Input: dimensioned drawing with shaded views. Units: mm. Origin: part minimum x, y, z. A direction names the side the tool comes from. Coordinates: 2 decimals unless noted, no trailing zeros. Order: outer loops, then holes, each group sorted by start corner. A loop starts at its lowest first (then second) coordinate and runs counter-clockwise, first axis right, second up. Notation, with made-up numbers: (-1.75, 70.25) -> (12.25, 70.25) arc R22 cw to (12.25, 91.25) -> close; hole circle Ø7 at (-17, 50). An arc over 180 degrees is marked (long way). Answer as CSV lines item,"result".
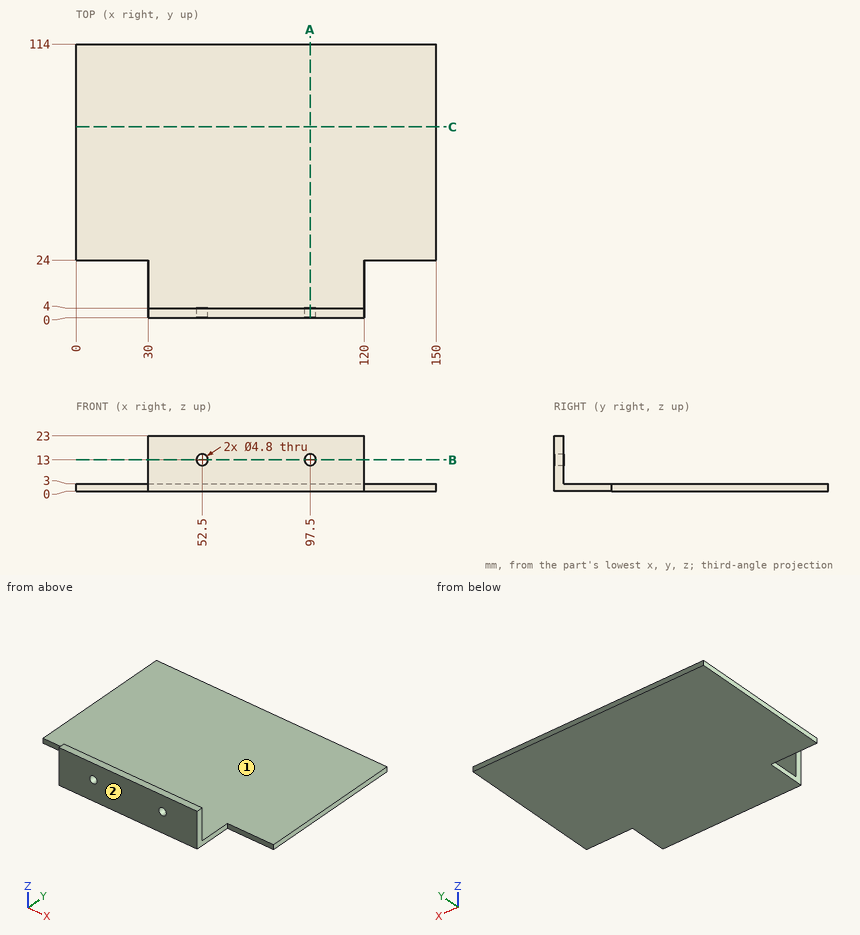
1. Cut plane C-C (y = 79.5). Return the cut outline in (x, z).
Findings:
outline,"(0, 0) -> (150, 0) -> (150, 3) -> (0, 3) -> close"
2. Contact query for flat-ended pins moving along their axis: pin 1 (12 mm diameter, centred on x = 75.5, z = 8.5, fed in from -Y); pin 2 (2.5 mm diameter, centred on x = 130.5, z = 1, fed in from -Y); pin 3 (1.5 mm diameter, centred on x = 91.5, z = 15, fed in from +Y); pin 4 (1 mm diameter, centred on x = 112.5, y = 24.5, fed in from +Z). Output: stop coordinate, or through.
Findings:
pin 1,"stops at y = 0"
pin 2,"stops at y = 24"
pin 3,"stops at y = 4"
pin 4,"stops at z = 3"
3. Ray query, line 1 along Z through (x, y) = (52.5, 3.1); line 2 along Y through (x, z) = (36, 9.75); line 3 along Z through (x, y) = (130.5, 93). Return the intervals inside material, ascending.
Findings:
line 1,"z = 0 to 10.6, 15.4 to 23"
line 2,"y = 0 to 4"
line 3,"z = 0 to 3"
4. Reachability of the marked faces 1 and 2 from +Z, -Z, +X, -X, +Y, -Y: full face, straight path, thin tool, end or side. Return the list, or none.
Findings:
face 1,"+Z, +X, -X, +Y"
face 2,"+Z, -Z, +X, -X, -Y"
5. Cut plane A-A (x = 97.5). Return the cut outline in (y, z).
Findings:
outline,"(0, 0) -> (114, 0) -> (114, 3) -> (4, 3) -> (4, 10.6) -> (0, 10.6) -> close; (0, 15.4) -> (4, 15.4) -> (4, 23) -> (0, 23) -> close"
6. Cut plane B-B (z = 13). Return the cut outline in (x, y), plus the area to 3 significant figures.
Findings:
outline,"(30, 0) -> (50.1, 0) -> (50.1, 4) -> (30, 4) -> close; (54.9, 0) -> (95.1, 0) -> (95.1, 4) -> (54.9, 4) -> close; (99.9, 0) -> (120, 0) -> (120, 4) -> (99.9, 4) -> close"
area,"322 mm2"
